```python
from build123d import *

# Parameters (mm, degrees)
SKETCH_1_W      = 40
SKETCH_1_H      = 16
EXTRUDE_1_DEPTH = 70
SKETCH_2_W      = 40
SKETCH_2_H      = 20
EXTRUDE_2_DEPTH = 220
SKETCH_4_W      = 200
SKETCH_4_H      = 250
EXTRUDE_4_DEPTH = 10


with BuildPart() as part:
    # 草图1 → 凸台-拉伸1 (new body)
    with BuildSketch(Plane(origin=(0, 0, 0), x_dir=(1, 0, 0), z_dir=(0, 1, 0))):
        Rectangle(SKETCH_1_W, SKETCH_1_H)
    extrude(amount=EXTRUDE_1_DEPTH)

    # 草图2 → 凸台-拉伸2 (add)
    with BuildSketch(Plane.XY.offset(8)):
        with Locations((0, 10)):
            Rectangle(SKETCH_2_W, SKETCH_2_H)
    extrude(amount=EXTRUDE_2_DEPTH)

    # 草图4 → 凸台-拉伸4 (add)
    with BuildSketch(Plane.XY.offset(228)):
        with Locations((-0.193037092, 69.445287213)):
            Rectangle(SKETCH_4_W, SKETCH_4_H)
    extrude(amount=EXTRUDE_4_DEPTH)


solid = part.part
```
Part model, mm, in its own coordinate system. A direction names the side the tool comes from. Round coordinates to 2 decimals unless told otherwise and drop trailing zeros. Loops run counter-clockwise (first coordinate to the right, second up) from the corner with the lowest first, then second, coordinate; pieces in that order, holes last.
Item 1: Cut at D-D, the plane x = -48. Give the cut face in (y, z), then the cut area to 3 significant figures.
Item 2: 3-axis set-ups, long thin cutter, end or side, ignore diameter. For faces 4 (the face through (0, 70, 0)), 5 (the face through (0, 45, 8)), 6 (the face through (20, 19, 82)), 7 (the face through (0, 0, 108)), 8 (the face through (-20, 19, 82)): which of +Z, -Z, +X, -X, +Y, -Y reach the whole face in a straight line?
Item 3: Drop flat-ended pins along their axis: P1, Ø12, axis at x = -5.5, z = 129, coming from the -Y side; P2, Ø5, axis at x = -3, y = 76.5, coming from the -Z side; P3, Ø8, axis at x = 2, z = 2, coming from the +Y side. Give the stop position or say it passes through.
Item 4: Cut at B-B, the plane y = 64.5. Give the cut face in (x, z).
Item 5: Cut at A-A, the plane y = 16.5. Give the cut face in (x, z), then the cut area to 3 significant figures.
Item 6: Drill centre lines: line 1 (Z direction, x = -69, y = 101.5); line 2 (X direction, y = 21, z = 3); line 3 (Y direction, x = 11, z = 217.5). Where is each one in solid material? Low to high.
Item 7: Mould opens along Z. For faces 1 (the face through (0, 35, -8)), 2 (the face through (0, 20, 116)), 3 (the face through (-100.193, 68, 233)) say: +Z half, -Z half, draft (parallel to the pull), parting line (faces both ways), or undercut.
Item 8: Cut at C-C, the plane z = 86. Give the cut face in (x, y).
A:
1. outline: (-55.55, 228) - (194.45, 228) - (194.45, 238) - (-55.55, 238) - close
1. area: 2,500 mm2
2. face 4: -Z, +X, -X, +Y
2. face 5: +X, -X, +Y
2. face 6: -Z, +X, +Y, -Y
2. face 7: -Z, +X, -X, -Y
2. face 8: -Z, -X, +Y, -Y
3. P1: stops at y = 0
3. P2: stops at z = 228
3. P3: stops at y = 70
4. outline: (-100.19, 228) - (99.81, 228) - (99.81, 238) - (-100.19, 238) - close; (-20, -8) - (20, -8) - (20, 8) - (-20, 8) - close
5. outline: (-100.19, 228) - (-20, 228) - (-20, -8) - (20, -8) - (20, 228) - (99.81, 228) - (99.81, 238) - (-100.19, 238) - close
5. area: 11,400 mm2
6. line 1: z = 228 to 238
6. line 2: x = -20 to 20
6. line 3: y = 0 to 20
7. face 1: -Z half
7. face 2: undercut
7. face 3: draft
8. outline: (-20, 0) - (20, 0) - (20, 20) - (-20, 20) - close
